from build123d import *

# Parameters (mm, degrees)
F1_DEPTH = 25
F2_R     = 3
F3_DEPTH = 25


with BuildPart() as f1:
    # F0 (on Front) → F1 (new body)
    with BuildSketch(Plane.XZ):
        Polygon((-58.138707, 3), (-58.138707, 0), (-38.138707, 0), (71.861293, 150), (70.341078, 153), (-39.658922, 3), align=None)
    extrude(amount=F1_DEPTH)

    # F2 (on Top) → F3 (cut)
    with BuildSketch(Plane.XY):
        with Locations((-48.138707, -12.5)):
            Circle(F2_R)
    extrude(amount=F3_DEPTH, mode=Mode.SUBTRACT)


solid = f1.part
Model file for the job. Use its own axes, mm. A direction names the side the tool comes from. Give positions to 0.01 mm unless a question says otherwise; leave off trailing zeros. Write each loop counter-clockwise with the first axis right and the second up, starting at its lowest first coordinate (ties: lowest second). Pieces come first, ordered by that corner, then holes. Notation, with made-up numbers: M -11.75,-16 L 46.25,-16 A26 ccw 46.25,16 Z; hole C 64.5,77.5 d9. An arc over 180 degrees is marked long. One line per item, written item: value. Start each with the question number.
Q1. Saw through at A-A, the plane y = -12.5. Write the cut outline in (x, z), plus the area to 3 significant figures.
Q2. Two-plate mould, pull along X, no slides. Class faces 1 (the cylindrical face through (-45.277, -11.599, 1.479)), 2 (the flat face through (16.11, -12.32, 79.05)), 3 (the flat face through (16, 0, 77)): +X half, -X half, draft (parallel to the pull), parting line (faces both ways), or undercut.
Q3. Saw through at C-C, the plane z = 60. Write the cut outline in (x, y).
Q4. 3-axis set-ups, long thin cutter, end or side, ignore diameter. For faces 4 (the flat face through (-51, -10, 3)), 5 (the flat face through (16.09, -12.32, 73.95)): which of +Z, -Z, +X, -X, +Y, -Y reach the whole face in a straight line?
Q5. Drop flat-ended pins along their axis: pin 1 Ø4 at (x, y) = (-20.5, -8) entering from -Z; pin 2 Ø12 at (x, y) = (58, -5) entering from +Z; pin 3 Ø4 at (y, z) = (-18.5, 115) entering from -X. Give the stop position or say it passes through.
Q6. Saw through at B-B, the plane y = -21. Write the cut outline in (x, z).
Q7. Probe probe 1 along X at (y, z) = (-12.5, 1.45); probe 2 along X at (y, z) = (-12.5, 1.85); probe 3 along Z at (x, y) = (48.5, -13.25). List the from-to ranges inside material, lowest first. Write a range as [from, to].
Q8. Saw through at D-D, the plane x = -3. Write the cut outline in (y, z).
Output values:
1. outline: M -58.14,0 L -51.14,0 L -51.14,3 L -58.14,3 Z; M -45.14,0 L -38.14,0 L 71.86,150 L 70.34,153 L -39.66,3 L -45.14,3 Z
1. area: 598 mm²
2. face 1: undercut
2. face 2: -X half
2. face 3: draft
3. outline: M 2.14,-25 L 5.86,-25 L 5.86,0 L 2.14,0 Z
4. face 4: +Z, -X, +Y, -Y
4. face 5: -Z, +X, +Y, -Y
5. pin 1: stops at z = 21.33
5. pin 2: stops at z = 144.35
5. pin 3: stops at x = 41.01
6. outline: M -58.14,0 L -38.14,0 L 71.86,150 L 70.34,153 L -39.66,3 L -58.14,3 Z
7. probe 1: x = [-58.14, -51.14], [-45.14, -37.08]
7. probe 2: x = [-58.14, -51.14], [-45.14, -36.78]
7. probe 3: z = [118.14, 123.22]
8. outline: M -25,47.92 L 0,47.92 L 0,52.99 L -25,52.99 Z
